Verification items for the finished model (mm, model axes). A direction names the side the tool comes from. Coordinates: 2 decimals unless noted, no trailing zeros. Order: outer loops, then holes, each group sorted by start corner. A loop starts at its lowest first (then second) coordinate and runs counter-clockwise, first axis right, second up. Notation, with made-up numbers: (61, 59) - (102, 59) arc R8 cw to (102, 63) - close; hole circle Ø9 at (35.25, -7). An arc over 180 degrees is marked (long way). One line per question, with ' | ' between items. Start each with the question number.
Autodesk Inventor part; units mm, degrees
ref_plane "Work Plane1" through (-15.0438, -15.0438, 25) normal (0, 0, -1) x (0, 1, 0)
ref_plane "YZ Plane" through (0, 0, 0) normal (1, 0, 0) x (0, 1, 0)
ref_plane "XZ Plane" through (0, 0, 0) normal (0, 1, 0) x (-1, 0, 0)
sketch "Sketch1" plane through (0, 0, 0) normal (0, 0, 1) x (1, 0, 0)
  arc A0 (-4.218, 13.0871) -> (12.3207, -6.1043) centre (0, 0) ccw
  circle A1 centre (0, 0) radius 14.25
  circle A2 centre (0, 0) radius 13
  point P0 (0, 0)
  dimension "d0" = 28.5
  dimension "d1" = 26
ref_plane "Work Plane1" through (-15.0438, -15.0438, 25) normal (0, 0, -1) x (0, 1, 0)
extrude "Extrusion1" add sketch "Sketch1" along normal up to surface (25 mm away)
sketch "Sketch2" plane through (0, 0, 25) normal (0, 0, 1) x (1, 0, 0)
  circle A0 centre (0, 0) radius 13.5
  circle A1 centre (0, 0) radius 13
  circle A2 centre (0, 0) radius 13
  dimension "d4" = 27
extrude "Extrusion2" add sketch "Sketch2" along normal blind 3
sketch "Sketch3" plane through (0, 0, 0) normal (0, 0, -1) x (-1, 0, 0)
  circle A0 centre (0, 0) radius 13
  circle A1 centre (0, 0) radius 13.5
  point P0 (0, 0)
extrude "Extrusion3" add sketch "Sketch3" along normal blind 3
properties part number "30_CUBE_openVCM_voicecoil"
Item 1: Gauge pin test, flat ends, axial feed: pin 1 (6 mm diameter, centred on x = -11.5, z = 24.5, fed in from -Y); pin 2 (8 mm diameter, centred on y = -6.5, z = 9, fed in from -X); pin 3 (1 mm diameter, centred on y = 3.5, z = 5.5, fed in from -X). Record the tip position at first contact, or that the pin passes through.
Item 2: Section check C-C (z = 12.5). Record the cut outline in (x, y).
Item 3: Set-up check for faces 1 (the cylindrical face through (13.163, 5.458, 12.325)), 2 (the flat face through (13, -5, 25)), 3 (the cylindrical face through (2.93, 13.18, -1.48)): record each of +Z, -Z, +X, -X, +Y, -Y from which the full face is reachable in a straight line by a thin tool's end or side.
Item 4: Thickness scan on probe 1 along X at (y, z) = (-0.5, 13.5); probe 2 along Y at (x, z) = (0, -0.9); probe 3 along Y at (x, z) = (0, 6). Record the ranges inside material, lowest first. Write a range as from..to.
Item 5: Section check A-A (y = 0). Record the cut outline in (x, z), then the cut area to 3 significant figures.
Item 6: Mould release check, pull along Z, two halves, no side actions. Record for faces 4 (the flat face through (-7.1, 11.1, 28)), 5 (the flat face through (7.1, 11.1, -3)), 6 (the cylindrical face through (-2.93, 13.18, 26.48)): +Z half, -Z half, draft (parallel to the pull), parting line (faces both ways), or undercut.
Completed:
1) pin 1: stops at y = -11.44 | pin 2: stops at x = -14.03 | pin 3: stops at x = -13.93
2) outline: circle Ø28.5 at (0, 0); hole circle Ø26 at (0, 0)
3) face 1: +Z, -Z | face 2: +Z | face 3: -Z
4) probe 1: x = -14.24..-12.99, 12.99..14.24 | probe 2: y = -13.5..-13, 13..13.5 | probe 3: y = -14.25..-13, 13..14.25
5) outline: (-14.25, 0) - (-13.5, 0) - (-13.5, -3) - (-13, -3) - (-13, 28) - (-13.5, 28) - (-13.5, 25) - (-14.25, 25) - close; (13, -3) - (13.5, -3) - (13.5, 0) - (14.25, 0) - (14.25, 25) - (13.5, 25) - (13.5, 28) - (13, 28) - close | area: 68.5 mm^2
6) face 4: +Z half | face 5: -Z half | face 6: draft
